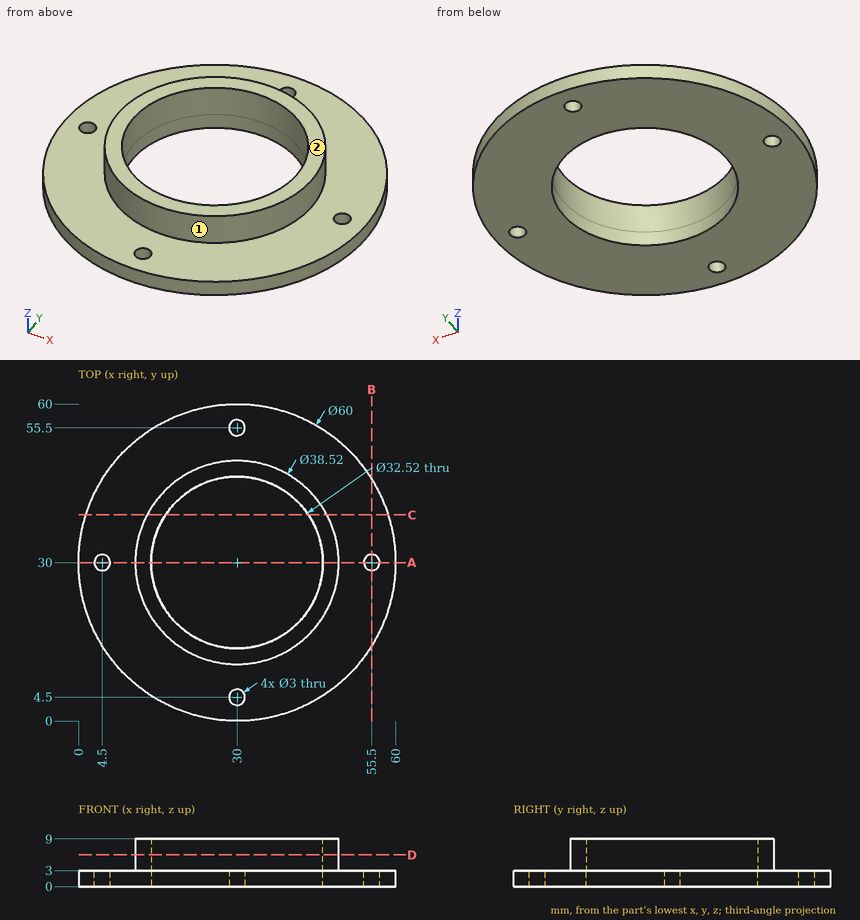
Job drawing, mm, ordinate dimensions from the low corner. One solid piece. A direction names the side the tool comes from. Round coordinates to 2 decimals unless told otherwise and drop trailing zeros. Order: outer loops, then holes, each group sorted by start corner. A loop starts at its lowest first (then second) coordinate and runs counter-clockwise, first axis right, second up. Notation, with made-up numbers: (-12.75, 78) -> (21.25, 78) arc R21 ccw to (21.25, 109) -> close; hole circle Ø2 at (-19.75, 86.5). An arc over 180 degrees is marked (long way). Answer in a Markdown table with one row per item.
1) Wall check: L1, parallel to Y at x = 30, z = 2.3; L2, parallel to Z at x = 57, y = 18.5; L3, parallel to Y at x = 30.5, z = 1. Give the ranges that are in metal, low to high.
Values:
| item | result |
|---|---|
| L1 | 0 to 3, 6 to 13.74, 46.26 to 54, 57 to 60 |
| L2 | 0 to 3 |
| L3 | 0 to 3.09, 5.91 to 13.75, 46.25 to 54.09, 56.91 to 60 |
2) Pin check, flat tips, straight feed: P1, Ø4, axis at x = 30, y = 4.5, coming from the +Z side; P2, Ø3, axis at y = 13, z = 5, coming from the -X side; P3, Ø3, axis at x = 19, z = 6, coming from the -Y side. Stop position of each tip, or through.
Values:
| item | result |
|---|---|
| P1 | z = 3 |
| P2 | x = 18.57 |
| P3 | y = 13.25 |
3) Band-saw the part on C-C on y = 39. Give the cut face in (x, z).
Values:
| item | result |
|---|---|
| outline | (1.38, 0) -> (16.46, 0) -> (16.46, 9) -> (12.97, 9) -> (12.97, 3) -> (1.38, 3) -> close; (43.54, 0) -> (58.62, 0) -> (58.62, 3) -> (47.03, 3) -> (47.03, 9) -> (43.54, 9) -> close |
4) Band-saw the part on A-A on y = 30. Give the cut face in (x, z).
Values:
| item | result |
|---|---|
| outline | (0, 0) -> (3, 0) -> (3, 3) -> (0, 3) -> close; (6, 0) -> (13.74, 0) -> (13.74, 9) -> (10.74, 9) -> (10.74, 3) -> (6, 3) -> close; (46.26, 0) -> (54, 0) -> (54, 3) -> (49.26, 3) -> (49.26, 9) -> (46.26, 9) -> close; (57, 0) -> (60, 0) -> (60, 3) -> (57, 3) -> close |
5) Band-saw the part on D-D on z = 6. Give the cut face in (x, y), and give its area (3 significant figures).
Values:
| item | result |
|---|---|
| outline | circle Ø38.52 at (30, 30); hole circle Ø32.52 at (30, 30) |
| area | 335 mm2 |
6) Which spindle directions (+Z, -Z, +X, -X, +Y, -Y) get a long thin tool onto all of the face, cutting with end or side? Do the marked faces 1 and 2. Say none if no direction does.
Values:
| item | result |
|---|---|
| face 1 | +Z |
| face 2 | +Z, +X, -X, +Y, -Y |
7) Band-saw the part on B-B on x = 55.5. Give the cut face in (y, z).
Values:
| item | result |
|---|---|
| outline | (14.2, 0) -> (28.5, 0) -> (28.5, 3) -> (14.2, 3) -> close; (31.5, 0) -> (45.8, 0) -> (45.8, 3) -> (31.5, 3) -> close |
